Source: CAD feature listing. Evaluate the final solid. Frame: model axes, mm. Face numbers are marked on the shaded views. A direction names the side the tool comes from. Give positions to 0.01 mm unless a question says otherwise; leave off trailing zeros. Write each loop counter-clockwise with the first axis right and the second up, starting at its lowest first coordinate (ties: lowest second). Pieces come first, ordered by that corner, then holes. Notation, with made-up numbers: M 37,35 L 47,35 A17 ccw 47,47 Z; hole C 37.5,14.25 d8. An arc over 180 degrees is marked long. Answer as a JSON object with one key per item and string values. Group by question number.
```python
from build123d import *

# Parameters (mm, degrees)
SKETCH_R     = 9.5
SKETCH_R_2   = 2.5
PAD_DEPTH    = 25
SKETCH001_R  = 4
POCKET_DEPTH = 12.5
CHAMFER_SIZE = 1


with BuildPart() as part:
    # Sketch → Pad (new body)
    with BuildSketch(Plane.XY):
        Circle(SKETCH_R)
        Circle(SKETCH_R_2, mode=Mode.SUBTRACT)
    extrude(amount=PAD_DEPTH)

    # Sketch001 (on Face4 of Pad) → Pocket (cut)
    with BuildSketch(Plane.XY.offset(25)):
        Circle(SKETCH001_R)
    extrude(amount=-POCKET_DEPTH, mode=Mode.SUBTRACT)

    # Chamfer
    chamfer_edges = [part.edges().sort_by_distance(p)[0] for p in [
        (-9.5, 0, 25),
        (-4, 0, 25),
        (-9.5, 0, 0),
        (-2.5, 0, 0),
    ]]
    chamfer(chamfer_edges, length=CHAMFER_SIZE)


solid = part.part
```
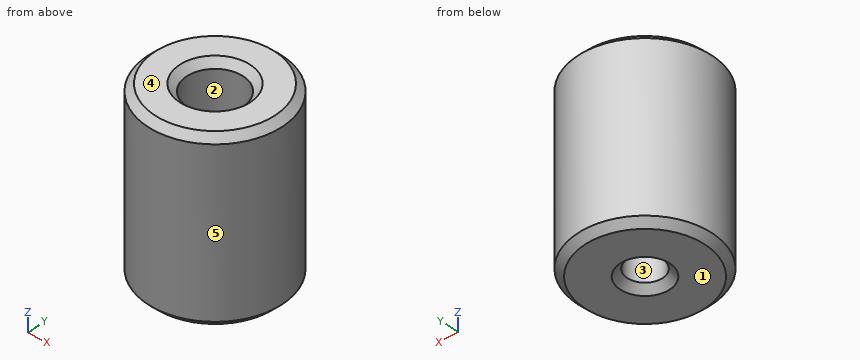
(1) Section D-D, the plane z = 20. Return loops of the section in (x, y).
(2) Section C-C, the plane z = 6.5. Return loops of the section in (x, y).
(3) Ray query, L1, parallel to X at y = -0.25, z = 20.75; L2, parallel to Y at x = 0, z = 9.5; L3, parallel to X at y = -2.5, z = 14.25. Return the intervals inside material, ascending. Write a range as [from, to].
(4) Contact query for flat-ended pins moving along their axis: pin 1 Ø5 at (x, z) = (-0.5, 13) entering from +Y; pin 2 Ø1 at (y, z) = (-1, 12) entering from -X; pin 3 Ø6.5 at (x, y) = (0, 0) entering from +Z; pin 4 Ø3 at (x, z) = (-3.5, 22) entering from +Y. Output: stop coordinate, or through.
(5) Section A-A, the plane x = 0. Return loops of the section in (y, z).
(6) Access query for the marked faces 1 and 2. Directions: +Z, -Z, +X, -X, +Y, -Y. A direction counts if a zero-diameter tool reaches every point of the face in a straight line with its end or side. Return the directions, or none.
(7) Pull-direction query (Y, two-part tool) for the marked faces 3, 4 and 5; classes: pulls with the +Y half, pulls with the -Y half, needs draft (parallel to the pull), parting line crosses it, or undercut.
Reported:
{
 "1": {"outline": "C 0,0 d19; hole C 0,0 d8"},
 "2": {"outline": "C 0,0 d19; hole C 0,0 d5"},
 "3": {"L1": "x = [-9.5, -3.99], [3.99, 9.5]", "L2": "y = [-9.5, -2.5], [2.5, 9.5]", "L3": "x = [-9.17, -3.12], [3.12, 9.17]"},
 "4": {"pin 1": "stops at y = 9.5", "pin 2": "stops at x = -9.49", "pin 3": "stops at z = 12.5", "pin 4": "stops at y = 9.29"},
 "5": {"outline": "M -9.5,1 L -8.5,0 L -3.5,0 L -2.5,1 L -2.5,12.5 L -4,12.5 L -4,24 L -5,25 L -8.5,25 L -9.5,24 Z; M 2.5,1 L 3.5,0 L 8.5,0 L 9.5,1 L 9.5,24 L 8.5,25 L 5,25 L 4,24 L 4,12.5 L 2.5,12.5 Z"},
 "6": {"face 1": "-Z, +X, -X, +Y, -Y", "face 2": "+Z"},
 "7": {"face 3": "undercut", "face 4": "needs draft", "face 5": "parting line crosses it"}
}
